Geometry check sheet. Reference: the model listing, model coordinates, mm. A direction names the side the tool comes from. Round coordinates to 2 decimals unless told otherwise and drop trailing zeros. Loops run counter-clockwise (first coordinate to the right, second up) from the corner with the lowest first, then second, coordinate; pieces in that order, holes last. Notation, with made-up numbers: (38.25, -4) - (50.25, -4) arc R21 cw to (50.25, 11) - close; hole circle Ø5 at (-10.75, 89.5). An arc over 180 degrees is marked (long way). Write item = value, one per line.
Autodesk Inventor part; units mm, degrees
ref_plane "YZ Plane" through (0, 0, 0) normal (1, 0, 0) x (0, 1, 0)
ref_plane "XZ Plane" through (0, 0, 0) normal (0, 1, 0) x (-1, 0, 0)
ref_plane "XY Plane" through (0, 0, 0) normal (0, 0, 1) x (1, 0, 0)
sketch "Esquisse1" plane through (0, 0, 0) normal (0, 0, 1) x (1, 0, 0)
  circle A0 centre (0, 0) radius 65
  dimension "d0" = 130
extrude "Extrusion1" add sketch "Esquisse1" along normal blind 79
sketch "Esquisse2" plane through (0, 0, 79) normal (0, 0, 1) x (1, 0, 0)
  circle A0 centre (0, 0) radius 74.5
  dimension "d3" = 149
extrude "Extrusion2" add sketch "Esquisse2" along normal blind 3
sketch "Esquisse3" plane through (0, 0, 82) normal (0, 0, 1) x (1, 0, 0)
  circle A0 centre (0, 0) radius 62.5
  dimension "d6" = 125
extrude "Extrusion3" cut sketch "Esquisse3" against normal blind 50.5
fillet "Congé1" radius 8 1 edges at (-65, 0, 0)
fillet "Congé2" radius 4 1 edges at (-65, 0, 79)
chamfer "Chanfrein1" distance 1.5 angle 60 1 edges at (-74.5, 0, 82) measured on face at (-31.6394, -62.7681, 82)
equation "\"nombredor\" = 1.61803"
equation "\"pi\" = 3.141593"
properties part number "Bol" material "Acier inoxydable"
(1) Section check D-D (z = 38). Enter the section's corners in (x, y).
Answers follow:
outline = circle Ø130 at (0, 0); hole circle Ø125 at (0, 0)
(2) Gauge pin test, flat ends, axial feed: pin 1 (2 mm diameter, centred on y = -38.5, z = 72.5, fed in from -X); pin 2 (12 mm diameter, centred on x = 39, z = 60, fed in from -Y); pin 3 (1 mm diameter, centred on y = 34, z = 36.5, fed in from +X). Record the tip position at first contact, or that the pin passes through.
Answers follow:
pin_1 = -53.09
pin_2 = -56
pin_3 = 55.7
(3) Scan lines: L1, parallel to Y at x = 0, z = 52; L2, parallel to Z at x = 17, y = 44; L3, parallel to X at y = -44, z = 47.5. Record each from-to range of solid material in increasing order. Write a range as [from, to].
Answers follow:
L1 = [-65, -62.5], [62.5, 65]
L2 = [0, 31.5]
L3 = [-47.84, -44.39], [44.39, 47.84]
(4) Section check A-A (y = 0). Enter the section's corners in (x, z), then the cut area to 3 significant figures.
Answers follow:
outline = (-74.5, 79) - (-69, 79) arc R4 cw to (-65, 75) - (-65, 8) arc R8 ccw to (-57, 0) - (57, 0) arc R8 ccw to (65, 8) - (65, 75) arc R4 cw to (69, 79) - (74.5, 79) - (74.5, 79.4) - (73, 82) - (62.5, 82) - (62.5, 31.5) - (-62.5, 31.5) - (-62.5, 82) - (-73, 82) - (-74.5, 79.4) - close
area = 4,380 mm²
(5) Mould release check, pull along X, two halves, no side actions. Record for faces 1 (the flat face through (54, 33, 82)), 2 (the conical face through (-9.52, -72.47, 81.84)), 3 (the cylindrical face through (-62.44, 2.75, 57.1)), 4 (the flat face through (-1, 1, 31.5)): pulls with the +X half, pulls with the -X half, needs draft (parallel to the pull), parting line crosses it, or undercut.
Answers follow:
face_1 = needs draft
face_2 = parting line crosses it
face_3 = undercut
face_4 = undercut
(6) Set-up check for faces 5 (the cylindrical face through (62, -19.52, 41.03)), 6 (the cylindrical face through (71.06, -22.38, 79.2)): record each of +Z, -Z, +X, -X, +Y, -Y from which the full face is reachable in a straight line by a thin tool's end or side.
Answers follow:
face_5 = -Z
face_6 = +Z, -Z
(7) Section check C-C (z = 26). Enter the section's corners in (x, y), then the cut area to 3 significant figures.
Answers follow:
outline = circle Ø130 at (0, 0)
area = 13,300 mm²
